Design review of the part built by this model. Coordinates are the model's own, in mm. A direction names the side the tool comes from. Give positions to 0.01 mm unless a question says otherwise; leave off trailing zeros. Answer as CSV lines item,"result".
from build123d import *
from build123d.topology import SkipClean

# Parameters (mm, degrees)
SKETCH1_R             = 1.9
SKETCH1_R_2           = 4.25
SKETCH1_R_3           = 1.1
BOSS_EXTRUDE1_DEPTH   = 5
SKETCH4_R             = 1.75
CUT_EXTRUDE3_DEPTH    = 2.25
CORTAR_EXTRUIR1_DEPTH = 10
REDONDEO1_R           = 10
REDONDEO3_R           = 1


with BuildPart() as part:
    # Sketch1 → Boss-Extrude1 (new body)
    with BuildSketch(Plane.XY):
        with BuildLine():
            Line((-18.926637777, 20.351096398), (-25.818616811, -18.423903602))
            ThreePointArc((-25.818616811, -18.423903602), (-14.988364044, -31.348903602), (-4.158111277, -18.423903602))
            Line((-4.158111277, -18.423903602), (-11.05009031, 20.351096398))
            ThreePointArc((-11.05009031, 20.351096398), (-14.988364044, 23.651096398), (-18.926637777, 20.351096398))
        make_face()
        with Locations((-14.988364044, 19.651096398)):
            Circle(SKETCH1_R, mode=Mode.SUBTRACT)
        with Locations((-14.988364044, -20.348903602)):
            Circle(SKETCH1_R_2, mode=Mode.SUBTRACT)
        with Locations((-6.988364044, -20.348903602)):
            Circle(SKETCH1_R_3, mode=Mode.SUBTRACT)
        with Locations((-9.331509794, -26.005757851)):
            Circle(SKETCH1_R_3, mode=Mode.SUBTRACT)
        with Locations((-14.988364044, -28.348903602)):
            Circle(SKETCH1_R_3, mode=Mode.SUBTRACT)
        with Locations((-20.645218293, -26.005757851)):
            Circle(SKETCH1_R_3, mode=Mode.SUBTRACT)
        with Locations((-22.988364044, -20.348903602)):
            Circle(SKETCH1_R_3, mode=Mode.SUBTRACT)
        with Locations((-20.645218293, -14.692049352)):
            Circle(SKETCH1_R_3, mode=Mode.SUBTRACT)
        with Locations((-14.988364044, -12.348903602)):
            Circle(SKETCH1_R_3, mode=Mode.SUBTRACT)
        with Locations((-9.331509794, -14.692049352)):
            Circle(SKETCH1_R_3, mode=Mode.SUBTRACT)
    extrude(amount=BOSS_EXTRUDE1_DEPTH)

    # Sketch4 → Cut-Extrude3 (cut)
    with BuildSketch(Plane(origin=(0, 0, 0), x_dir=(-1, 0, 0), z_dir=(0, 0, -1))):
        with Locations((22.988364044, -20.348903602)):
            Circle(SKETCH4_R)
        with Locations((20.645218293, -26.005757851)):
            Circle(SKETCH4_R)
        with Locations((14.988364044, -28.348903602)):
            Circle(SKETCH4_R)
        with Locations((9.331509794, -26.005757851)):
            Circle(SKETCH4_R)
        with Locations((6.988364044, -20.348903602)):
            Circle(SKETCH4_R)
        with Locations((9.331509794, -14.692049352)):
            Circle(SKETCH4_R)
        with Locations((14.988364044, -12.348903602)):
            Circle(SKETCH4_R)
        with Locations((20.645218293, -14.692049352)):
            Circle(SKETCH4_R)
    extrude(amount=-CUT_EXTRUDE3_DEPTH, mode=Mode.SUBTRACT)

    # Croquis1 → Cortar-Extruir1 (cut)
    with SkipClean():  # the faces are left unmerged after this step: merging them gives an invalid solid
        with BuildSketch(Plane(origin=(0, 0, 0), x_dir=(-1, 0, 0), z_dir=(0, 0, -1))):
            with BuildLine():
                Line((11.003110402, 19.994248567), (8.279982388, -11.631242473))
                ThreePointArc((8.279982388, -11.631242473), (5.584323122, -14.642414809), (4.158111277, -18.423903602))
                Line((4.158111277, -18.423903602), (11.05009031, 20.351096398))
                ThreePointArc((11.05009031, 20.351096398), (11.022584598, 20.173201167), (11.003110402, 19.994248567))
            make_face()
        extrude(amount=-CORTAR_EXTRUIR1_DEPTH, mode=Mode.SUBTRACT)

    # Redondeo1
    redondeo1_edges = [part.edges().sort_by_distance(p)[0] for p in [
        (-8.279982388, -11.631242473, 2.5),
    ]]
    fillet(redondeo1_edges, radius=REDONDEO1_R)

    # Redondeo3
    redondeo3_edges = [part.edges().sort_by_distance(p)[0] for p in [
        (-14.988364044, -31.348903602, 5),
        (-9.795996729, 5.975237179, 5),
        (-7.906176898, -10.910629635, 5),
        (-14.988364044, 23.651096398, 5),
        (-22.372627294, 0.963596398, 5),
    ]]
    fillet(redondeo3_edges, radius=REDONDEO3_R)


solid = part.part
Q1. To check wall thickness, follow probe 1 along X at (y, z) = (-26.5, 3.6); probe 2 along X at (y, z) = (-15, 0.5); probe 3 along X at (y, z) = (-21, 3). State the ranges of each line that lie inside material, in increasing order. Write a range as from..to.
Filled sheet:
probe 1,"x = -24.11..-21.63, -19.66..-10.31, -8.35..-5.87"
probe 2,"x = -25.21..-22.37, -18.92..-11.05, -7.61..-5.38"
probe 3,"x = -25.97..-23.87, -22.1..-19.19, -10.79..-7.87, -6.1..-4.01"
Q2. We need section A-A, the plane z = 1.65. State how many separate pieces and enclosed holes the cut face has, and give its area (3 significant figures).
Filled sheet:
separate pieces,"1"
enclosed holes,"10"
area,"628 mm^2"
Q3. The part is to be moulded in two halves that separate along X. For faces 1 (the flat face through (-15, -9, 5)), 2 (the flat face through (-22.324, 1.235, 1.972)), 3 (the cylindrical face through (-13.233, 18.923, 2.465)), say which applies: pulls with the +X half, pulls with the -X half, needs draft (parallel to the pull), parting line crosses it, or undercut.
Filled sheet:
face 1,"needs draft"
face 2,"pulls with the -X half"
face 3,"undercut"
Q4. For faces 4 (the cylindrical face through (-9.1, -24.27, 1.11)), 5 (the cylindrical face through (-8.315, -15.113, 3.606)), list the 3-axis set-ups (+Z, -Z, +X, -X, +Y, -Y) from which the entire face can be reached by the end or side of a thin tool; tool diameter is ignored.
Filled sheet:
face 4,"-Z"
face 5,"+Z, -Z"
Q5. Clearance check with flat-ended pins moving along their axes: pin 1 Ø1 at (y, z) = (9.5, 2) entering from -X; pin 2 Ø1.5 at (x, z) = (-16, 1) entering from +Y; pin 3 Ø3 at (x, y) = (-9.33, -26.01) entering from -Z. State where each tip first meets the part, or that it passes through.
Filled sheet:
pin 1,"stops at x = -20.94"
pin 2,"stops at y = 23.64"
pin 3,"stops at z = 2.25"
